Geometry: final body of the model. Coordinates: model frame, mm. Face numbers are marked on the shaded views. A direction names the side the tool comes from. Coordinates: 2 decimals unless noted, no trailing zeros. Write each loop counter-clockwise with the first axis right and the second up, starting at its lowest first coordinate (ties: lowest second). Pieces come first, ordered by that corner, then holes. Notation, with made-up numbers: (-28, 76) -> (-19, 76) arc R21 ccw to (-19, 83) -> close; hole circle Ø3 at (1, 7.5). An arc over 180 degrees is marked (long way). One line per item, written item: value.
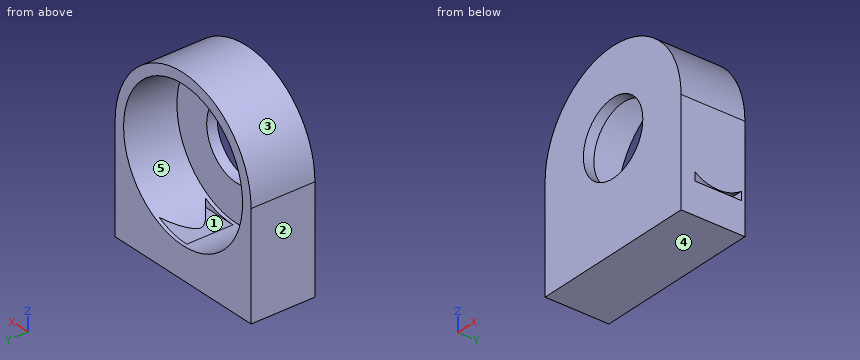
```python
from build123d import *

# Parameters (mm, degrees)
F0_R      = 35
F1_DEPTH  = 25.4
F3_DEPTH  = 25
F5_DEPTH  = 40
F6_R      = 17.5
F7_DEPTH  = 5
F8_DEPTH  = 5
F9_W      = 80
F9_H      = 25
F10_DEPTH = 25


with BuildPart() as f1:
    # F0 (on Front) → F1 (new body)
    with BuildSketch(Plane.XZ):
        with BuildLine():
            Line((40, -50), (40, 0))
            ThreePointArc((40, 0), (0, 40), (-40, 0))
            Line((-40, 0), (-40, -50))
            Line((-40, -50), (40, -50))
        make_face()
        Circle(F0_R, mode=Mode.SUBTRACT)
    extrude(amount=F1_DEPTH)

    # F2 (on face) → F3 (join)
    with BuildSketch(Plane.XZ.offset(25.4)):
        with BuildLine():
            Line((-40, -25), (-40, -50))
            Line((-40, -50), (40, -50))
            Line((40, -50), (40, -25))
            Line((40, -25), (24.4948974278, -25))
            ThreePointArc((24.4948974278, -25), (0, -35), (-24.4948974278, -25))
            Line((-24.4948974278, -25), (-40, -25))
        make_face()
        with BuildLine():
            Line((24.4948974278, -25), (-24.4948974278, -25))
            ThreePointArc((-24.4948974278, -25), (0, -35), (24.4948974278, -25))
        make_face()
    extrude(amount=F3_DEPTH)

    # F4 (on face) → F5 (cut)
    with BuildSketch(Plane.YZ.offset(40)):
        with BuildLine():
            Line((-23.7, -35), (-1.7, -35))
            Line((-1.7, -35), (-1.7, -31))
            ThreePointArc((-1.7, -31), (-12.7, -34.6), (-23.7, -31))
            Line((-23.7, -31), (-23.7, -35))
        make_face()
    extrude(amount=-F5_DEPTH, mode=Mode.SUBTRACT)

    # F6 (on face) → F7 (join)
    with BuildSketch(Plane.XZ.offset(25.4)):
        with BuildLine():
            Line((-40, 0), (-40, -25))
            Line((-40, -25), (40, -25))
            Line((40, -25), (40, 0))
            ThreePointArc((40, 0), (0, 40), (-40, 0))
        make_face()
        Circle(F6_R, mode=Mode.SUBTRACT)
    extrude(amount=F7_DEPTH)

    # F8 (add): a face of the model
    f8_faces = [f1.faces().sort_by_distance(p)[0] for p in [
        (0, -50.4, -37.5),
    ]]
    extrude(f8_faces, amount=F8_DEPTH)

    # F9 (on face) → F10 (cut)
    with BuildSketch(Plane.XY.offset(-25)):
        with Locations((0, -42.9)):
            Rectangle(F9_W, F9_H)
    extrude(amount=-F10_DEPTH, mode=Mode.SUBTRACT)


solid = f1.part
```
(1) Line query: line 1 (Z direction, x = 0, y = -15); line 2 (Z direction, x = 0, y = -29); line 3 (X direction, y = -10.5, z = -0.5). Output: solid intervals per line, ascending. Write a range as [from, to].
Responses:
line 1: z = [-50, -35], [35, 40]
line 2: z = [-50, -17.5], [17.5, 40]
line 3: x = [-40, -35], [35, 40]
(2) Section A-A (x = 13.5). Return the cut outline in (y, z), then the cut area to 3 significant figures.
Responses:
outline: (-30.4, -50) -> (0, -50) -> (0, -32.29) -> (-1.7, -32.29) -> (-1.7, -35) -> (-23.7, -35) -> (-23.7, -32.29) -> (-25.4, -32.29) -> (-25.4, -11.14) -> (-30.4, -11.14) -> close; (-30.4, 11.14) -> (-25.4, 11.14) -> (-25.4, 32.29) -> (0, 32.29) -> (0, 37.65) -> (-30.4, 37.65) -> close; (-21.68, -32.29) arc R18.61 ccw to (-3.72, -32.29) -> close
area: 881 mm2
(3) Reachability of the marked faces 4 and 5 from +Z, -Z, +X, -X, +Y, -Y: full face, straight path, thin tool, end or side. Return the list, or none.
Responses:
face 4: -Z, +X, -X, +Y, -Y
face 5: +Y
(4) Pull-direction query (Z, two-part tool) for the marked faces 1, 2 and 3; classes: released by +Z, released by -Z, zero draft, split by the parting line, or undercut.
Responses:
face 1: undercut
face 2: zero draft
face 3: released by +Z
(5) Section B-B (z = -3). Return the cut outline in (x, y).
Responses:
outline: (-40, -30.4) -> (-17.24, -30.4) -> (-17.24, -25.4) -> (-34.87, -25.4) -> (-34.87, 0) -> (-40, 0) -> close; (17.24, -30.4) -> (40, -30.4) -> (40, 0) -> (34.87, 0) -> (34.87, -25.4) -> (17.24, -25.4) -> close
(6) Section C-C (x = -9.5). Return the cut outline in (y, z).
Responses:
outline: (-30.4, -50) -> (0, -50) -> (0, -33.69) -> (-25.4, -33.69) -> (-25.4, -14.7) -> (-30.4, -14.7) -> close; (-30.4, 14.7) -> (-25.4, 14.7) -> (-25.4, 33.69) -> (0, 33.69) -> (0, 38.86) -> (-30.4, 38.86) -> close
(7) Section D-D (z = 20.5). Return the cut outline in (x, y), then the cut area to 3 significant figures.
Responses:
outline: (-34.35, -30.4) -> (34.35, -30.4) -> (34.35, 0) -> (28.37, 0) -> (28.37, -25.4) -> (-28.37, -25.4) -> (-28.37, 0) -> (-34.35, 0) -> close
area: 647 mm2
(8) First-contact query: pin 1 (4 mm diameter, centred on x = -10.5, y = -9.5, fed in from +Z); pin 2 (6 mm diameter, centred on x = 9.5, y = -21.5, fed in from +Z); pin 3 (11 mm diameter, centred on x = 15, y = -12, fed in from +Z). Flat tips, straight axial feed; report the tip coordinate or a pass-through.
Responses:
pin 1: stops at z = 39.09
pin 2: stops at z = 39.47
pin 3: stops at z = 38.86
